from build123d import *

# Parameters (mm, degrees)
PAD_DEPTH       = 12
POCKET_DEPTH    = 62
SKETCH019_W     = 31
SKETCH019_H     = 21.780884
POCKET002_DEPTH = 17
SKETCH020_R     = 2
POCKET003_DEPTH = 4
CYLINDER_R      = 4
CYLINDER_DEPTH  = 28
POCKET032_DEPTH = 5
SKETCH084_W     = 7.885986
SKETCH084_H     = 7.189331
PAD020_DEPTH    = 0.5
POCKET038_DEPTH = 100


with BuildPart() as part:
    # Sketch010 → Pad (new body, symmetric)
    with BuildSketch(Plane.XY):
        with BuildLine():
            Line((12.639868, 59.984547), (-12.639868, 59.984547))
            Line((-12.639868, 59.984547), (-17.867889, 82.058411))
            Line((-17.867889, 82.058411), (-17.867889, 102.222236))
            ThreePointArc((-15.867889, 104.222236), (-17.282103, 103.63645), (-17.867889, 102.222236))
            Line((-15.867889, 104.222236), (-8.154342, 104.222236))
            ThreePointArc((-7.154342, 103.222236), (-7.447235, 103.929343), (-8.154342, 104.222236))
            Line((-7.154342, 103.222236), (-7.154342, 92.189331))
            Line((-7.154342, 92.189331), (7.154342, 92.189331))
            Line((7.154342, 92.189331), (7.154342, 103.222236))
            ThreePointArc((8.154342, 104.222236), (7.447235, 103.929343), (7.154342, 103.222236))
            Line((8.154342, 104.222236), (15.867889, 104.222236))
            ThreePointArc((17.867889, 102.222236), (17.282103, 103.63645), (15.867889, 104.222236))
            Line((17.867889, 102.222236), (17.867889, 82.058411))
            Line((17.867889, 82.058411), (12.639868, 59.984547))
        make_face()
    extrude(amount=PAD_DEPTH, both=True)

    # Sketch011 → Pocket (cut)
    with BuildSketch(Plane.XZ.offset(-54)):
        Polygon((0, 13.813917), (-22.117895, 13.813917), (-22.117895, -0.189388), (-22.117895, -17.743416), (0, -17.743416), (22.658901, -17.743416), (22.658901, -0.111897), (22.658901, 13.813917), align=None)
        Polygon((-18.596464, 0), (-18.596464, 5.287208), (-8.154342, 8), (-7.443202, 8.179805), (0, 8.179805), (7.519913, 8.179805), (8.154342, 8), (18.531284, 5.287208), (18.531284, -0.112287), (18.531284, -5.399495), (8.154342, -8), (7.554242, -8.253323), (0.11104, -8.253323), (-7.443202, -8.253323), (-8.154342, -8), (-18.596464, -5.371119), align=None, mode=Mode.SUBTRACT)
    extrude(amount=-POCKET_DEPTH, mode=Mode.SUBTRACT)

    # Sketch019 → Pocket002 (cut)
    with BuildSketch(Plane.XY.offset(0.8)):
        with Locations((0.01352, 95.005211)):
            Rectangle(SKETCH019_W, SKETCH019_H)
    extrude(amount=-POCKET002_DEPTH, mode=Mode.SUBTRACT)

    # Sketch020 → Pocket003 (cut)
    with BuildSketch(Plane.XY.offset(0.8)):
        with Locations((-11.1, 94.9)):
            Circle(SKETCH020_R)
        with Locations((11.3, 94.9)):
            Circle(SKETCH020_R)
        with Locations((0.013518, 88.3)):
            Circle(SKETCH020_R)
    extrude(amount=POCKET003_DEPTH, mode=Mode.SUBTRACT)

    # Cylinder → Cylinder (cut)
    with BuildSketch(Plane.XZ.offset(-85)):
        Circle(CYLINDER_R)
    extrude(amount=CYLINDER_DEPTH, mode=Mode.SUBTRACT)

    # Sketch067 → Pocket032 (cut)
    with BuildSketch(Plane.XY.offset(7)):
        Polygon((-7.9, 83), (0, 68), (7.9, 83), (0, 98), align=None)
    extrude(amount=POCKET032_DEPTH, mode=Mode.SUBTRACT)

    # Sketch084 → Pad020 (join)
    with BuildSketch(Plane.XY.offset(0.8)):
        with Locations((-0.023809, 88.594665)):
            Rectangle(SKETCH084_W, SKETCH084_H)
    extrude(amount=PAD020_DEPTH)

    # Sketch085 → Groove (revolve, cut)
    with BuildSketch(Plane.XY):
        with BuildLine():
            ThreePointArc((9.252061, 79.708405), (10.164814, 75.624968), (11.720768, 71.740822))
            Line((11.720768, 71.740822), (11.720768, 58.4589))
            Line((11.720768, 58.4589), (0, 58.4589))
            Line((0, 58.4589), (0, 79.708405))
            Line((9.252061, 79.708405), (0, 79.708405))
        make_face()
    revolve(axis=Axis((0, 0, 0), (0, 1, 0)), mode=Mode.SUBTRACT)

    # Sketch089 → Pocket038 (cut)
    with BuildSketch(Plane.XZ):
        Polygon((-2.5, 0.8), (0, 3.3), (2.5, 0.8), align=None)
    extrude(amount=-POCKET038_DEPTH, mode=Mode.SUBTRACT)


solid = part.part
Source: CAD feature listing. Evaluate the final solid. Frame: model axes, mm. A direction names the side the tool comes from. Round coordinates to 2 decimals unless told otherwise and drop trailing zeros. Loops run counter-clockwise (first coordinate to the right, second up) from the corner with the lowest first, then second, coordinate; pieces in that order, holes last.
Q1. Mould query, pull axis Z, two halves, no side actions, for faces 1 (the face through (-17.27, 103.65, 0.05)), 2 (the face through (6, 91, 8.18)), 3 (the face through (13.079, 76.878, -6.766)), 4 (the face through (2, 79.708, -4)). Classes: pulls with the +Z half, pulls with the -Z half, needs draft (parallel to the pull), parting line crosses it, or undercut.
Q2. Section C-C, the plane y = 76.5. Return loops of the section in (x, z), plus the area to 3 significant figures.
Q3. Section D-D, the plane y = 66. Return loops of the section in (x, z).
Q4. Access query for faces 5 (the face through (-1, 85, 3)), 6 (the face through (-5.446, 87.659, 7.582)), 7 (the face through (10, 92, 0.8)), 8 (the face through (1.86, 87.53, 3.41)). Directions: +Z, -Z, +X, -X, +Y, -Y. A direction counts if a zero-diameter tool reaches every point of the face in a straight line with its end or side. Return the directions, or none.
Q5. Ray query, line 1 (X direction, y = 88.3, z = 3.8); line 2 (X direction, y = 83.1, z = 0); line 3 (Z direction, x = 0, y = 83.05). Return the intervals inside material, ascending.
Q6. First-contact query: P1, Ø4.5, axis at x = 11.3, y = 94.9, coming from the -Z side; P2, Ø2.5, axis at x = 0.01, y = 88.3, coming from the +Z side; P3, Ø8, axis at x = 2.5, z = 5.5, coming from the +Y side; P4, Ø4, axis at x = -3.5, y = 75.5, coming from the -Z side. Flat tips, straight axial feed; report the tip coordinate or a pass-through.
Q7. Section A-A, the plane y = 94.9. Return loops of the section in (x, z), plus the area to 3 significant figures.
Q8. Section B-B, the plane z = 0. Return loops of the section in (x, y), plus the area to 3 significant figures.
Solutions:
1. face 1: needs draft
1. face 2: pulls with the +Z half
1. face 3: pulls with the -Z half
1. face 4: undercut
2. outline: (-16.55, -5.89) - (-8.15, -8) - (-7.44, -8.25) - (-5.49, -8.25) arc R9.91 cw to (-5.6, 8.18) - (-7.44, 8.18) - (-8.15, 8) - (-16.55, 5.82) - close; (5.49, -8.25) - (7.55, -8.25) - (8.15, -8) - (16.55, -5.9) - (16.55, 5.8) - (8.15, 8) - (7.52, 8.18) - (5.6, 8.18) arc R9.91 cw to start
2. area: 217 mm2
3. outline: (-14.06, -6.51) - (-8.69, -7.87) arc R11.72 cw to (-8.7, 7.86) - (-14.06, 6.46) - close; (8.69, -7.87) - (14.06, -6.52) - (14.06, 6.45) - (8.7, 7.86) arc R11.72 cw to start
4. face 5: -Z, -Y
4. face 6: +Z
4. face 7: -Z, +Y
4. face 8: -Z
5. line 1: x = -17.87 to -1.99, 2.01 to 17.87
5. line 2: x = -17.87 to -4, 4 to 17.87
5. line 3: z = -8.25 to -4, 4 to 7
6. P1: stops at z = 0.8
6. P2: stops at z = 7
6. P3: stops at y = 92.19
6. P4: passes through
7. outline: (-17.87, -5.55) - (-15.49, -6.15) - (-15.49, 0.8) - (-13.1, 0.8) - (-13.1, 4.8) - (-9.1, 4.8) - (-9.1, 0.8) - (-7.15, 0.8) - (-7.15, 8.18) - (-7.44, 8.18) - (-8.15, 8) - (-17.87, 5.48) - close; (7.15, 0.8) - (9.3, 0.8) - (9.3, 4.8) - (13.3, 4.8) - (13.3, 0.8) - (15.51, 0.8) - (15.51, -6.16) - (17.87, -5.57) - (17.87, 5.46) - (8.15, 8) - (7.52, 8.18) - (7.15, 8.18) - close
7. area: 129 mm2
8. outline: (-17.87, 82.06) - (-12.64, 59.98) - (-11.72, 59.98) - (-11.72, 71.74) arc R26 ccw to (-9.25, 79.71) - (-4, 79.71) - (-4, 84.11) - (-15.49, 84.11) - (-15.49, 104.22) - (-15.87, 104.22) arc R2 ccw to (-17.87, 102.22) - close; (4, 79.71) - (9.25, 79.71) arc R26 ccw to (11.72, 71.74) - (11.72, 59.98) - (12.64, 59.98) - (17.87, 82.06) - (17.87, 102.22) arc R2 ccw to (15.87, 104.22) - (15.51, 104.22) - (15.51, 84.11) - (4, 84.11) - close
8. area: 366 mm2
